CAD build for the part. Positions are in the model's coordinates, mm. A direction names the side the tool comes from. Coordinates: 2 decimals unless noted, no trailing zeros. Order: outer loops, then holes, each group sorted by start corner. A loop starts at its lowest first (then second) coordinate and runs counter-clockwise, first axis right, second up. Notation, with made-up numbers: (-32, 33) - (13, 33) arc R24 ccw to (13, 50) - close; hole circle Ø7 at (-36, 56). An arc over 180 degrees is marked (long way). Return JSON: item names as keys, results as strings.
from build123d import *

# Parameters (mm, degrees)
BOSS_EXTRUDE1_DEPTH = 6


with BuildPart() as part:
    # Sketch1 → Boss-Extrude1 (new body)
    with BuildSketch(Plane(origin=(0, 0, 0), x_dir=(1, 0, 0), z_dir=(0, 0, -1))):
        with BuildLine():
            Line((-27.759328596, 44.902453019), (-0.000594147, 0.000961069))
            Line((-0.000594147, 0.000961069), (27.758140303, 44.902453019))
            ThreePointArc((27.758140303, 44.902453019), (19.099343857, 67.218890553), (-0.000594147, 52.790082274))
            ThreePointArc((-0.000594147, 52.790082274), (-19.10053215, 67.218890553), (-27.759328596, 44.902453019))
        make_face()
        with BuildLine():
            Line((23.50522882, 47.531662771), (-0.000594147, 9.509521573))
            Line((-0.000594147, 9.509521573), (-23.506417113, 47.531662771))
            ThreePointArc((-23.506417113, 47.531662771), (-20.25901365, 61.29590524), (-6.49477118, 58.048501777))
            Line((-6.49477118, 58.048501777), (-0.000594147, 47.543763589))
            Line((-0.000594147, 47.543763589), (6.493582887, 58.048501777))
            ThreePointArc((6.493582887, 58.048501777), (20.257825357, 61.29590524), (23.50522882, 47.531662771))
        make_face(mode=Mode.SUBTRACT)
    extrude(amount=BOSS_EXTRUDE1_DEPTH)


solid = part.part
Item 1: Mould opens along Y. For faces 1 (the flat face through (-11.589, -28.254, -2.958)), 2 (the flat face through (-14.074, -22.766, -2.958)), 3 (the flat face through (0, -52, -6)) say: released by +Y, released by -Y, zero draft, split by the parting line, or undercut.
Findings below:
{"face 1": "undercut", "face 2": "released by +Y", "face 3": "zero draft"}
Item 2: Band-saw the part on A-A, the plane x = 13. List the corners of the cut face in (y, z), then the cut area to 3 significant figures.
Findings below:
{"outline": "(-67.66, -6) - (-62.59, -6) - (-62.59, 0) - (-67.66, 0) - close; (-30.54, -6) - (-21.03, -6) - (-21.03, 0) - (-30.54, 0) - close", "area": "87.5 mm²"}
Item 3: Band-saw the part on B-B, the plane y = -38.5. List the corners of the cut face in (x, z).
Findings below:
{"outline": "(-23.8, -6) - (-17.92, -6) - (-17.92, 0) - (-23.8, 0) - close; (17.92, -6) - (23.8, -6) - (23.8, 0) - (17.92, 0) - close"}
Item 4: Wall check: L1, parallel to Y at x = -15, z = -3.1; L2, parallel to Y at x = 4.5, z = -1.5; L3, parallel to X at y = -44, z = -2.75. Give the ranges that are in metal, low to high. Write a range as [from, to].
Findings below:
{"L1": "y = [-67.79, -62.79], [-33.77, -24.26]", "L2": "y = [-63.5, -54.82], [-16.79, -7.28]", "L3": "x = [-27.2, -21.32], [21.32, 27.2]"}
Item 5: Drop flat-ended pins along their axis: P1, Ø1, axis at y = -43.5, z = -1, coming from the +X side; P2, Ø1.5, axis at x = -15.5, z = -4.5, coming from the +Y side; P3, Ø1.5, axis at y = -30.5, z = -3, coming from the +X side. Give the stop position or say it passes through.
Findings below:
{"P1": "stops at x = 27.2", "P2": "stops at y = -23.86", "P3": "stops at x = 19.32"}
Item 6: Band-saw the part on D-D, the plane z = -4.25. List the corners of the cut face in (x, y).
Findings below:
{"outline": "(-27.76, -44.9) arc R15 ccw (long way) to (0, -52.79) arc R15 ccw (long way) to (27.76, -44.9) - (0, 0) - close; hole (-23.51, -47.53) arc R10 ccw to (-6.49, -58.05) - (0, -47.54) - (6.49, -58.05) arc R10 ccw to (23.51, -47.53) - (0, -9.51) - close"}
Item 7: Which spindle directions (+Z, -Z, +X, -X, +Y, -Y) get a long thin tool onto all of the face, cutting with end or side? Do faces 4 (the flat face through (11.92, -28.79, -2.96)), 5 (the flat face through (0, -52, 0)). Say none if no direction does.
Findings below:
{"face 4": "+Z, -Z", "face 5": "+Z, +X, -X, +Y, -Y"}
Item 8: Band-saw the part on C-C, the plane y = -60.5. List the corners of the cut face in (x, z).
Findings below:
{"outline": "(-27.87, -6) - (-21.37, -6) - (-21.37, 0) - (-27.87, 0) - close; (-8.63, -6) - (-2.13, -6) - (-2.13, 0) - (-8.63, 0) - close; (2.13, -6) - (8.63, -6) - (8.63, 0) - (2.13, 0) - close; (21.37, -6) - (27.87, -6) - (27.87, 0) - (21.37, 0) - close"}
